```python
from build123d import *

# Parameters (mm, degrees)
ESQUISSE1_R                  = 9.9
BOSS_EXTRU_1_DEPTH           = 1.75
ESQUISSE2_R                  = 3.5
ESQUISSE2_R_2                = 2.475
BOSS_EXTRU_2_DEPTH           = 2.1
ESQUISSE3_R                  = 2.725
ESQUISSE3_R_2                = 2.225
BOSS_EXTRU_3_DEPTH           = 0.3
ESQUISSE4_R                  = 0.95
ENL_V_MAT_EXTRU_1_DEPTH      = 15.520416661
ESQUISSE5_R                  = 0.6
ENL_V_MAT_EXTRU_2_DEPTH      = 15.520416661
R_P_TITION_CIRCULAIRE1_COUNT = 4


with BuildPart() as part:
    # Esquisse1 → Boss.-Extru.1 (new body)
    with BuildSketch(Plane(origin=(0, 0, 0), x_dir=(1, 0, 0), z_dir=(0, 1, 0))):
        with Locations(Location((0, 0, 0), (0, 0, 270))):
            Circle(ESQUISSE1_R)
    extrude(amount=BOSS_EXTRU_1_DEPTH)

    # Esquisse2 → Boss.-Extru.2 (add)
    with BuildSketch(Plane(origin=(0, 1.75, 0), x_dir=(1, 0, 0), z_dir=(0, 1, 0))):
        with Locations(Location((0, 0, 0), (0, 0, 270))):
            Circle(ESQUISSE2_R)
        with Locations(Location((0, 0, 0), (0, 0, 270))):
            Circle(ESQUISSE2_R_2, mode=Mode.SUBTRACT)
    extrude(amount=BOSS_EXTRU_2_DEPTH)

    # Esquisse3 → Boss.-Extru.3 (add)
    with BuildSketch(Plane.XZ):
        with Locations(Location((0, 0, 0), (0, 0, 90))):
            Circle(ESQUISSE3_R)
        with Locations(Location((0, 0, 0), (0, 0, 270))):
            Circle(ESQUISSE3_R_2, mode=Mode.SUBTRACT)
    extrude(amount=BOSS_EXTRU_3_DEPTH)

    # Esquisse4 → Enlèv. mat.-Extru.1 (cut, through all)
    with BuildSketch(Plane.XZ):
        with Locations(Location((0, 0, 0), (0, 0, 270))):
            Circle(ESQUISSE4_R)
    extrude(amount=-ENL_V_MAT_EXTRU_1_DEPTH, mode=Mode.SUBTRACT)

    # Esquisse5 → Enlèv. mat.-Extru.2 (cut, through all)
    with BuildSketch(Plane.XZ):
        with Locations(Location((0, 4.5, 0), (0, 0, 270))):
            Circle(ESQUISSE5_R)
        with Locations(Location((0, 6.5, 0), (0, 0, 270))):
            Circle(ESQUISSE5_R)
        with Locations(Location((0, 8.5, 0), (0, 0, 270))):
            Circle(ESQUISSE5_R)
    enl_v_mat_extru_2 = extrude(amount=-ENL_V_MAT_EXTRU_2_DEPTH, mode=Mode.SUBTRACT)

    # Répétition circulaire1: Enlèv. mat.-Extru.2 ×4 about axis
    r_p_tition_circulaire1_axis = Axis((0, 0, 0), (0, 1, 0))
    for i in range(1, R_P_TITION_CIRCULAIRE1_COUNT):
        add(enl_v_mat_extru_2.rotate(r_p_tition_circulaire1_axis, i * 360 / R_P_TITION_CIRCULAIRE1_COUNT), mode=Mode.SUBTRACT)


solid = part.part
```
The listing builds one solid part. Answer for the finished solid, in the listing's coordinates (mm). A direction names the side the tool comes from. Coordinates: 2 decimals unless noted, no trailing zeros. Write each loop counter-clockwise with the first axis right and the second up, starting at its lowest first coordinate (ties: lowest second). Pieces come first, ordered by that corner, then holes.
Q1. Section B-B, the plane z = 4.5 is taken. Write down the section's boundary in (x, y), then the cut area to 3 significant figures.
Returned:
outline: (-8.82, 0) - (-0.6, 0) - (-0.6, 1.75) - (-8.82, 1.75) - close; (0.6, 0) - (8.82, 0) - (8.82, 1.75) - (0.6, 1.75) - close
area: 28.8 mm2
Q2. Given P1, Ø1, axis at y = 2.5, z = 1, coming from the -X side; P2, Ø2, axis at x = 3.5, z = 3, coming from the +Y side; P3, Ø10, axis at x = 2, z = 7.5, coming from the +Y side; P4, Ø4, axis at x = 0, z = 0, coming from the -Y side, each flat-ended and moving along its own axis, determine where each tip first touches the part or whether it passes through.
Returned:
P1: stops at x = -3.46
P2: stops at y = 1.75
P3: stops at y = 3.85
P4: stops at y = 0
Q3. The mould has two halves that part along Z. Classify faces 4 (the cylindrical face through (2.974, 0.863, 9.443)), 5 (the cylindrical face through (-7.1, 0.9, 0)), 6 (the flat face through (-2, 3.85, 2)): released by +Z, released by -Z, zero draft, split by the parting line, or undercut.
Returned:
face 4: split by the parting line
face 5: undercut
face 6: zero draft
Q4. Which of the six approach directions +Z, -Z, +X, -X, +Y, -Y give full straight-line access (tool end or side, diameter ignored) to faces 1 (the cylindrical face through (0, 0.9, 5.1)), 2 (the flat face through (-2.1, 0, 2.1)), 3 (the flat face through (0, 1.75, 1.1))?
Returned:
face 1: +Y, -Y
face 2: -Y
face 3: +Y
Q5. Find the intervals of material crossed by line 1 along X through (y, z) = (2.6, 0) (3 decimals); line 2 along Y through (x, z) = (-2.5, -6.25); line 3 along X through (y, z) = (3.55, -1), in increasing order.
Returned:
line 1: x = -3.5 to -2.475, 2.475 to 3.5
line 2: y = 0 to 1.75
line 3: x = -3.35 to -2.26, 2.26 to 3.35
Q6. Section D-D, the plane y = 2.1 is taken. Write down the section's boundary in (x, z) (3 decimals).
Returned:
outline: circle Ø7 at (0, 0); hole circle Ø4.95 at (0, 0)
Q7. Section A-A, the plane y = 0.45 is taken. Give the number of separate pieces and of enclosed holes in the cut face, then the cut area to 4 significant figures.
Returned:
separate pieces: 1
enclosed holes: 13
area: 291.5 mm2
Q8. Section C-C, the plane x = -6.5 is taken. Write down the section's boundary in (y, z), then the cut area to 3 significant figures.
Returned:
outline: (0, -7.47) - (1.75, -7.47) - (1.75, -0.6) - (0, -0.6) - close; (0, 0.6) - (1.75, 0.6) - (1.75, 7.47) - (0, 7.47) - close
area: 24.0 mm2
